from build123d import *

# Parameters (mm, degrees)
SCHIZZO1_R                   = 13
SCHIZZO1_R_2                 = 2.5
SCHIZZO1_R_3                 = 4
SCHIZZO1_R_4                 = 1.5
SCHIZZO1_R_5                 = 8
ESTRUSIONE_ESTRUSIONE1_DEPTH = 10
SCHIZZO2_W                   = 30
SCHIZZO2_H                   = 120
TAGLIO_ESTRUSIONE1_DEPTH     = 2


with BuildPart() as part:
    # Schizzo1 → Estrusione-Estrusione1 (new body)
    with BuildSketch(Plane.XY):
        Polygon((2, 0), (448, 0), (450, 2), (450, 118), (448, 120), (2, 120), (0, 118), (0, 2), align=None)
        with Locations((225, 60)):
            Circle(SCHIZZO1_R, mode=Mode.SUBTRACT)
        with Locations(Location((246.213203436, 81.213203436, 0), (0, 0, 180))):
            Circle(SCHIZZO1_R_2, mode=Mode.SUBTRACT)
        with Locations((390, 100)):
            Circle(SCHIZZO1_R_3, mode=Mode.SUBTRACT)
        with Locations((246.213203436, 38.786796564)):
            Circle(SCHIZZO1_R_2, mode=Mode.SUBTRACT)
        with Locations(Location((203.786796564, 38.786796564, 0), (0, 0, 180))):
            Circle(SCHIZZO1_R_2, mode=Mode.SUBTRACT)
        with Locations(Location((60, 100, 0), (0, 0, 180))):
            Circle(SCHIZZO1_R_3, mode=Mode.SUBTRACT)
        with Locations((15, 30)):
            Circle(SCHIZZO1_R_4, mode=Mode.SUBTRACT)
        with Locations(Location((435, 30, 0), (0, 0, 180))):
            Circle(SCHIZZO1_R_4, mode=Mode.SUBTRACT)
        with Locations((203.786796564, 81.213203436)):
            Circle(SCHIZZO1_R_2, mode=Mode.SUBTRACT)
        with Locations((435, 90)):
            Circle(SCHIZZO1_R_4, mode=Mode.SUBTRACT)
        with Locations(Location((15, 90, 0), (0, 0, 180))):
            Circle(SCHIZZO1_R_4, mode=Mode.SUBTRACT)
        with Locations((310, 80)):
            Circle(SCHIZZO1_R_5, mode=Mode.SUBTRACT)
        with BuildLine():
            Line((330.75, 108.5), (330.75, 98.5))
            ThreePointArc((330.75, 98.5), (333.5, 95.75), (336.25, 98.5))
            Line((336.25, 98.5), (336.25, 108.5))
            ThreePointArc((336.25, 108.5), (333.5, 111.25), (330.75, 108.5))
        make_face(mode=Mode.SUBTRACT)
        with BuildLine():
            Line((289.25, 108.5), (289.25, 98.5))
            ThreePointArc((289.25, 98.5), (286.5, 95.75), (283.75, 98.5))
            Line((283.75, 98.5), (283.75, 108.5))
            ThreePointArc((283.75, 108.5), (286.5, 111.25), (289.25, 108.5))
        make_face(mode=Mode.SUBTRACT)
        with BuildLine():
            Line((330.75, 51.5), (330.75, 61.5))
            ThreePointArc((330.75, 61.5), (333.5, 64.25), (336.25, 61.5))
            Line((336.25, 61.5), (336.25, 51.5))
            ThreePointArc((336.25, 51.5), (333.5, 48.75), (330.75, 51.5))
        make_face(mode=Mode.SUBTRACT)
        with BuildLine():
            Line((289.25, 51.5), (289.25, 61.5))
            ThreePointArc((289.25, 61.5), (286.5, 64.25), (283.75, 61.5))
            Line((283.75, 61.5), (283.75, 51.5))
            ThreePointArc((283.75, 51.5), (286.5, 48.75), (289.25, 51.5))
        make_face(mode=Mode.SUBTRACT)
    extrude(amount=-ESTRUSIONE_ESTRUSIONE1_DEPTH)

    # Schizzo2 → Taglio-Estrusione1 (cut)
    with BuildSketch(Plane.XY):
        with Locations((15, 60)):
            Rectangle(SCHIZZO2_W, SCHIZZO2_H)
        with Locations((615.438855383, 60)):
            Rectangle(SCHIZZO2_W, SCHIZZO2_H)
    extrude(amount=-TAGLIO_ESTRUSIONE1_DEPTH, mode=Mode.SUBTRACT)


solid = part.part
Input: part model. Units: mm. Frame: model coordinates. A direction names the side the tool comes from. Give positions to 0.01 mm unless a question says otherwise; leave off trailing zeros. Order: outer loops, then holes, each group sorted by start corner. A loop starts at its lowest first (then second) coordinate and runs counter-clockwise, first axis right, second up. Notation, with made-up numbers: (-18, 64.5) - (-2, 64.5) arc R12 cw to (-2, 87.5) - close; hole circle Ø3 at (88, 89.25). An arc over 180 degrees is marked (long way). Answer as a JSON object with one key per item and string values. Group by question number.
Q1. Cut plane A-A, the plane x = 60. Output: boundary loops of the cut face in (y, z).
Q2. Cut plane C-C, the plane x = 220. Output: boundary loops of the cut face in (y, z).
Q3. Mould query, pull axis X, two halves, no side actions, for faces 1 (the face through (283.75, 57, -5)), 2 (the face through (450, 59, -5)), 3 (the face through (228, 120, -5)). Classes: pulls with the +X half, pulls with the -X half, needs draft (parallel to the pull), parting line crosses it, or undercut.
Q4. Cut plane D-D, the plane z = -8.5. Count the separate pieces of the cut face and the enclosed holes in it, then the cut area to 3 significant figures.
Q5. Cut plane B-B, the plane y = 56. Output: boundary loops of the cut face in (x, z), then the cut area to 3 significant figures.
Q6. Set-up query: faces 4 (the face through (15, 61, -2)), 5 (the face through (289.25, 104, -5)), 6 (the face through (222, 0, -5)). Return all of +Z, -Z, +X, -X, +Y, -Y with unobstructed straight access to the full face (end or side cutting, diameter ignored); none if empty.
Q7. Line query: probe 1 along Y at (x, z) = (435, -2.75); probe 2 along X at (y, z) = (90, -4.75); probe 3 along X at (y, z) = (106, -4). Output: solid intervals per line, ascending.
Q8. First-contact query: pin 1 Ø3 at (x, y) = (246.21, 81.21) entering from +Z; pin 2 Ø3.5 at (x, y) = (15, 90) entering from +Z. Flat tips, straight axial feed; report the tip coordinate or a pass-through.
Results:
{
 "1": {"outline": "(0, -10) - (96, -10) - (96, 0) - (0, 0) - close; (104, -10) - (120, -10) - (120, 0) - (104, 0) - close"},
 "2": {"outline": "(0, -10) - (48, -10) - (48, 0) - (0, 0) - close; (72, -10) - (120, -10) - (120, 0) - (72, 0) - close"},
 "3": {"face 1": "undercut", "face 2": "pulls with the +X half", "face 3": "needs draft"},
 "4": {"separate pieces": "1", "enclosed holes": "16", "area": "52,700 mm^2"},
 "5": {"outline": "(0, -10) - (212.63, -10) - (212.63, 0) - (30, 0) - (30, -2) - (0, -2) - close; (237.37, -10) - (283.75, -10) - (283.75, 0) - (237.37, 0) - close; (289.25, -10) - (330.75, -10) - (330.75, 0) - (289.25, 0) - close; (336.25, -10) - (450, -10) - (450, 0) - (336.25, 0) - close", "area": "4,080 mm^2"},
 "6": {"face 4": "+Z, -X, +Y, -Y", "face 5": "+Z, -Z", "face 6": "+Z, -Z, +X, -X, -Y"},
 "7": {"probe 1": "0 to 28.5, 31.5 to 88.5, 91.5 to 120", "probe 2": "0 to 13.5, 16.5 to 433.5, 436.5 to 450", "probe 3": "0 to 283.75, 289.25 to 330.75, 336.25 to 450"},
 "8": {"pin 1": "through", "pin 2": "z = -2"}
}
